The listing builds one solid part. Answer for the finished solid, in the listing's coordinates (mm). A direction names the side the tool comes from. Give positions to 0.01 mm unless a question says otherwise; leave off trailing zeros. Write each loop counter-clockwise with the first axis right and the second up, starting at its lowest first coordinate (ties: lowest second). Pieces come first, ordered by that corner, then holes. Notation, with made-up numbers: (-17.5, 40) - (-7.5, 40) arc R18 ccw to (-7.5, 47) - close; hole circle Ø4 at (-33.5, 28). An arc over 180 degrees is marked (long way). One line per question, with ' | ' between items. Start each with the question number.
1. A cutting plane is placed at B-B (z = 1). Determine the outline of the cut face in (x, y).
2. A cutting plane is placed at D-D (z = 26.5). Determine the outline of the cut face in (x, y).
3. Find the intervals of material crossed by L1, parallel to Z at x = -13, y = -11.45; L2, parallel to X at y = -11.4, z = 3.5; L3, parallel to X at y = -13.05, z = 28, in increasing order. Write a range as from..to.
4. The mould has two halves that part along Z. Classify faces 4 (the face through (41.5, -12.54, -37.07)), 5 (the face through (37.035, -12.465, -34.614)), 6 (the face through (-21.046, -12.535, 23.626)), 7 (the face through (-1, -15, 1)): +Z half, -Z half, draft (parallel to the pull), parting line (faces both ways), or undercut.
5. Given P1, Ø1.5, axis at x = -15.5, y = -12, coming from the -Z side; P2, Ø4, axis at x = -13, z = -6.5, coming from the -Y side; P3, Ø1, axis at x = 24, y = -13, coming from the -Z side, each flat-ended and moving along its own axis, determine where each tip first touches the part or whether it passes through.
6. A cutting plane is placed at C-C (y = -13.3). State how many separate pieces and enclosed holes the cut face has, then the cut area to 3 significant figures.
7. A cutting plane is placed at A-A (x = -33). Determine the outline of the cut face in (y, z).
8. For faces 1 (the face through (0, -12, 5)), 2 (the face through (-30, -12, 23.5)), 3 (the face through (-10, -12, -18.5)), determine the directions among +Z, -Z, +X, -X, +Y, -Y from which every point of the face is accessible in a straight line to the end or side of a thin tool.
```python
from build123d import *

# Parameters (mm, degrees)
F1_R     = 2.1
F1_R_2   = 1.6
F1_R_3   = 3.05
F1_W     = 23
F1_H     = 21.447819
F2_DEPTH = 5
F3_R     = 5


with BuildPart() as f2:
    # F1 (on offset) → F2 (new body)
    with BuildSketch(Plane.XZ.offset(10)):
        Polygon((23, -18.5), (23, -38.5), (43, -38.5), (43, 38.5), (9.512293, 38.5), (-21, 23.5), (-43, 23.5), (-43, -18.5), align=None)
        with Locations((-33, -6.5)):
            Circle(F1_R, mode=Mode.SUBTRACT)
        with Locations((-13, -6.5)):
            Circle(F1_R, mode=Mode.SUBTRACT)
        with Locations((27.253961, -34.684543)):
            Circle(F1_R_2, mode=Mode.SUBTRACT)
        with Locations((38.63319, -34.684543)):
            Circle(F1_R_2, mode=Mode.SUBTRACT)
        with Locations((35, -9.5)):
            Circle(F1_R_3, mode=Mode.SUBTRACT)
        with Locations((-33, 13.5)):
            Circle(F1_R, mode=Mode.SUBTRACT)
        with Locations((-13, 13.5)):
            Circle(F1_R, mode=Mode.SUBTRACT)
        with Locations((11.5, 4.606424)):
            Rectangle(F1_W, F1_H, mode=Mode.SUBTRACT)
        with Locations((9.512293, 26.5)):
            Circle(F1_R_3, mode=Mode.SUBTRACT)
        with Locations((35, 30.5)):
            Circle(F1_R_3, mode=Mode.SUBTRACT)
    extrude(amount=F2_DEPTH)

    # F3
    f3_edges = [f2.edges().sort_by_distance(p)[0] for p in [
        (-43, -12.5, -18.5),
        (-43, -12.5, 23.5),
        (0, -12.5, -6.117485),
        (0, -12.5, 15.330334),
        (23, -12.5, 15.330334),
        (23, -12.5, -6.117485),
        (23, -12.5, -18.5),
        (23, -12.5, -38.5),
        (43, -12.5, -38.5),
        (43, -12.5, 38.5),
        (-21, -12.5, 23.5),
        (9.512293, -12.5, 38.5),
    ]]
    fillet(f3_edges, radius=F3_R)


solid = f2.part
```
Determined:
1) outline: (-43, -15) - (0, -15) - (0, -10) - (-43, -10) - close; (23, -15) - (43, -15) - (43, -10) - (23, -10) - close
2) outline: (-14.9, -15) - (6.46, -15) - (6.46, -10) - (-14.9, -10) - close; (12.56, -15) - (43, -15) - (43, -10) - (12.56, -10) - close
3) L1: -18.5..-8.6, -4.4..11.4, 15.6..27.43 | L2: -43..0, 23..43 | L3: -11.85..6.86, 12.17..33.25, 36.75..43
4) face 4: -Z half | face 5: undercut | face 6: +Z half | face 7: draft
5) P1: z = -18.5 | P2: through | P3: z = -37.07
6) separate pieces: 1 | enclosed holes: 10 | area: 4,090 mm2
7) outline: (-15, -18.5) - (-10, -18.5) - (-10, -8.6) - (-15, -8.6) - close; (-15, -4.4) - (-10, -4.4) - (-10, 11.4) - (-15, 11.4) - close; (-15, 15.6) - (-10, 15.6) - (-10, 23.5) - (-15, 23.5) - close
8) face 1: +Y, -Y | face 2: +Z, -X, +Y, -Y | face 3: -Z, -X, +Y, -Y
